```python
from build123d import *

# Parameters (mm, degrees)
F0_W     = 130.7084
F0_H     = 50.8
F1_DEPTH = 1.524
F2_R     = 2.0955
F3_DEPTH = 25.4
F4_R     = 2.54
F6_DEPTH = 25.4


with BuildPart() as f1:
    # F0 (on Top) → F1 (new body)
    with BuildSketch(Plane.XY):
        Polygon((-73.3806, -52.578), (73.3806, -52.578), (73.3806, -33.528), (92.4306, -33.528), (92.4306, 31.115), (73.533, 31.115), (73.533, 49.5554), (63.6905, 49.5554), (63.6905, 82.6135), (-63.6905, 82.6135), (-63.6905, 49.5554), (-73.533, 49.5554), (-73.533, 31.115), (-92.4306, 31.115), (-92.4306, -33.528), (-73.3806, -33.528), align=None)
        Rectangle(F0_W, F0_H, mode=Mode.SUBTRACT)
    extrude(amount=F1_DEPTH)

    # F2 (on face) → F3 (cut)
    with BuildSketch(Plane.XY.offset(1.524)):
        with Locations((69.6341, -27.8511)):
            Circle(F2_R)
        with Locations((69.6341, 27.4447)):
            Circle(F2_R)
        with Locations((-69.6341, 27.4447)):
            Circle(F2_R)
        with Locations((-69.6341, -27.8511)):
            Circle(F2_R)
    extrude(amount=-F3_DEPTH, mode=Mode.SUBTRACT)

    # F4
    f4_edges = [f1.edges().sort_by_distance(p)[0] for p in [
        (63.6905, 82.6135, 0.762),
        (-63.6905, 82.6135, 0.762),
    ]]
    fillet(f4_edges, radius=F4_R)

    # F5 (on face) → F6 (cut)
    with BuildSketch(Plane.XY.offset(1.524)):
        with BuildLine():
            Line((53.7083, 67.488136), (53.7083, 74.854136))
            ThreePointArc((53.7083, 74.854136), (51.100731, 77.634491), (48.376736, 74.9681))
            Line((48.376736, 74.9681), (48.376736, 67.6021))
            ThreePointArc((48.376736, 67.6021), (50.986741, 64.935709), (53.7083, 67.488136))
        make_face()
        with BuildLine():
            ThreePointArc((-53.7083, 67.551636), (-50.986741, 64.999209), (-48.376736, 67.6656))
            Line((-48.376736, 67.6656), (-48.376736, 75.0316))
            ThreePointArc((-48.376736, 75.0316), (-51.100731, 77.697991), (-53.7083, 74.917636))
            Line((-53.7083, 74.917636), (-53.7083, 67.551636))
        make_face()
    extrude(amount=-F6_DEPTH, mode=Mode.SUBTRACT)


solid = f1.part
```
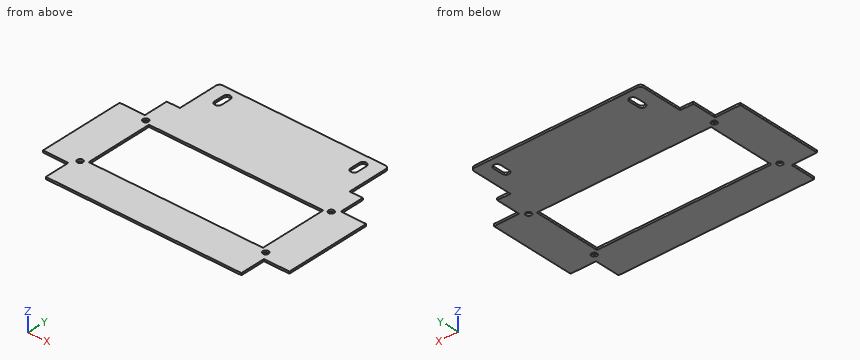
Design review of the part built by this model. Coordinates are the model's own, in mm. Coordinates: 2 decimals unless noted, no trailing zeros. Loops run counter-clockwise (first coordinate to the right, second up) from the corner with the lowest first, then second, coordinate; pieces in that order, holes last. Notation, with made-up numbers: M 33,72.25 L 70,72.25 A16 ccw 70,80.25 Z; hole C 42,11.25 d9. An arc over 180 degrees is marked long. One line per question, with ' | ' between items.
(1) We need section B-B (x = 10). Give the boundary of the cut face in (y, z), and give its area (3 significant figures).
Filled in:
outline: M -52.58,0 L -25.4,0 L -25.4,1.52 L -52.58,1.52 Z; M 25.4,0 L 82.61,0 L 82.61,1.52 L 25.4,1.52 Z | area: 129 mm^2
(2) We need section A-A (y = 23.5). Give the boundary of the cut face in (x, z).
Filled in:
outline: M -92.43,0 L -65.35,0 L -65.35,1.52 L -92.43,1.52 Z; M 65.35,0 L 92.43,0 L 92.43,1.52 L 65.35,1.52 Z
(3) We need section C-C (y = 69.5). Give the boundary of the cut face in (x, z), and give its area (3 significant figures).
Filled in:
outline: M -63.69,0 L -53.71,0 L -53.71,1.52 L -63.69,1.52 Z; M -48.38,0 L 48.38,0 L 48.38,1.52 L -48.38,1.52 Z; M 53.71,0 L 63.69,0 L 63.69,1.52 L 53.71,1.52 Z | area: 178 mm^2
(4) For pin 1 Ø0.5 at (y, z) = (37, 1) entering from -X; pin 2 Ø0.5 at (y, z) = (71, 1) entering from +X; pin 3 Ø3.5 at (x, y) = (-69.63, 27.44) entering from +Z; pin 4 Ø0.8 at (y, z) = (62.5, 1) entering from -X, all flat-tipped, find the tip position at first contact; note any pin that passes through.
Filled in:
pin 1: stops at x = -73.53 | pin 2: stops at x = 63.69 | pin 3: passes through | pin 4: stops at x = -63.69
(5) We need section D-D (x = -50.5). Give the boundary of the cut face in (y, z).
Filled in:
outline: M -52.58,0 L -25.4,0 L -25.4,1.52 L -52.58,1.52 Z; M 25.4,0 L 65.05,0 L 65.05,1.52 L 25.4,1.52 Z; M 77.64,0 L 82.61,0 L 82.61,1.52 L 77.64,1.52 Z
(6) Wall thickness on probe 1 along Y at (x, z) = (-23, 1.05); probe 2 along X at (y, z) = (69.5, 0.5); probe 3 along X at (y, z) = (13.5, 1.3): over which ranges is each line inside the solid? List them lowest first.
Filled in:
probe 1: y = -52.58 to -25.4, 25.4 to 82.61 | probe 2: x = -63.69 to -53.71, -48.38 to 48.38, 53.71 to 63.69 | probe 3: x = -92.43 to -65.35, 65.35 to 92.43
